```python
from build123d import *

# Parameters (mm, degrees)
Y_KSEKLIK_EKSTR_ZYON1_DEPTH = 40
RADYUS1_R                   = 1
RADYUS2_R                   = 0.3
RADYUS3_R                   = 1


with BuildPart() as part:
    # Çizim1 → Yükseklik-Ekstrüzyon1 (new body)
    with BuildSketch(Plane.XY):
        with BuildLine():
            Line((-8.6, -3.2), (-9.7, -3.2))
            Line((-9.7, -3.2), (-9.7, -3.7))
            Line((-9.7, -3.7), (-10, -3.7))
            Line((-10, -3.7), (-10, -10))
            Line((-10, -10), (-3.7, -10))
            Line((-3.7, -10), (-3.7, -9.7))
            Line((-3.7, -9.7), (-3.2, -9.7))
            Line((-3.2, -9.7), (-3.2, -8.6))
            Line((-3.2, -8.6), (-7.610050506, -8.6))
            Line((-7.610050506, -8.6), (-2.217957246, -3.20790674))
            ThreePointArc((-2.217957246, -3.20790674), (-1.299073648, -3.677282646), (-0.289258242, -3.889258242))
            Line((-0.289258242, -3.889258242), (0, -3.6))
            Line((0, -3.6), (0.289258242, -3.889258242))
            ThreePointArc((0.289258242, -3.889258242), (1.299073648, -3.677282646), (2.217957246, -3.20790674))
            Line((2.217957246, -3.20790674), (7.610050506, -8.6))
            Line((7.610050506, -8.6), (3.2, -8.6))
            Line((3.2, -8.6), (3.2, -9.7))
            Line((3.2, -9.7), (3.7, -9.7))
            Line((3.7, -9.7), (3.7, -10))
            Line((3.7, -10), (10, -10))
            Line((10, -10), (10, -3.7))
            Line((10, -3.7), (9.7, -3.7))
            Line((9.7, -3.7), (9.7, -3.2))
            Line((9.7, -3.2), (8.6, -3.2))
            Line((8.6, -3.2), (8.6, -7.610050506))
            Line((8.6, -7.610050506), (3.20790674, -2.217957246))
            ThreePointArc((3.20790674, -2.217957246), (3.677282646, -1.299073648), (3.889258242, -0.289258242))
            Line((3.889258242, -0.289258242), (3.6, 0))
            Line((3.6, 0), (3.889258242, 0.289258242))
            ThreePointArc((3.889258242, 0.289258242), (3.677282646, 1.299073648), (3.20790674, 2.217957246))
            Line((3.20790674, 2.217957246), (8.6, 7.610050506))
            Line((8.6, 7.610050506), (8.6, 3.2))
            Line((8.6, 3.2), (9.7, 3.2))
            Line((9.7, 3.2), (9.7, 3.7))
            Line((9.7, 3.7), (10, 3.7))
            Line((10, 3.7), (10, 10))
            Line((10, 10), (3.7, 10))
            Line((3.7, 10), (3.7, 9.7))
            Line((3.7, 9.7), (3.2, 9.7))
            Line((3.2, 9.7), (3.2, 8.6))
            Line((3.2, 8.6), (7.610050506, 8.6))
            Line((7.610050506, 8.6), (2.217957246, 3.20790674))
            ThreePointArc((2.217957246, 3.20790674), (1.299073648, 3.677282646), (0.289258242, 3.889258242))
            Line((0.289258242, 3.889258242), (0, 3.6))
            Line((0, 3.6), (-0.289258242, 3.889258242))
            ThreePointArc((-0.289258242, 3.889258242), (-1.299073648, 3.677282646), (-2.217957246, 3.20790674))
            Line((-2.217957246, 3.20790674), (-7.610050506, 8.6))
            Line((-7.610050506, 8.6), (-3.2, 8.6))
            Line((-3.2, 8.6), (-3.2, 9.7))
            Line((-3.2, 9.7), (-3.7, 9.7))
            Line((-3.7, 9.7), (-3.7, 10))
            Line((-3.7, 10), (-10, 10))
            Line((-10, 10), (-10, 3.7))
            Line((-10, 3.7), (-9.7, 3.7))
            Line((-9.7, 3.7), (-9.7, 3.2))
            Line((-9.7, 3.2), (-8.6, 3.2))
            Line((-8.6, 3.2), (-8.6, 7.610050506))
            Line((-8.6, 7.610050506), (-3.20790674, 2.217957246))
            ThreePointArc((-3.20790674, 2.217957246), (-3.677282646, 1.299073648), (-3.889258242, 0.289258242))
            Line((-3.889258242, 0.289258242), (-3.6, 0))
            Line((-3.6, 0), (-3.889258242, -0.289258242))
            ThreePointArc((-3.889258242, -0.289258242), (-3.677282646, -1.299073648), (-3.20790674, -2.217957246))
            Line((-3.20790674, -2.217957246), (-8.6, -7.610050506))
            Line((-8.6, -7.610050506), (-8.6, -3.2))
        make_face()
        with BuildLine():
            Line((1.967124912, -1.542860843), (2.333452378, -1.909188309))
            ThreePointArc((2.333452378, -1.909188309), (2.333452378, -2.333452378), (1.909188309, -2.333452378))
            Line((1.909188309, -2.333452378), (1.542860843, -1.967124912))
            ThreePointArc((1.542860843, -1.967124912), (0, -2.5), (-1.542860843, -1.967124912))
            Line((-1.542860843, -1.967124912), (-1.909188309, -2.333452378))
            ThreePointArc((-1.909188309, -2.333452378), (-2.333452378, -2.333452378), (-2.333452378, -1.909188309))
            Line((-2.333452378, -1.909188309), (-1.967124912, -1.542860843))
            ThreePointArc((-1.967124912, -1.542860843), (-2.5, 0), (-1.967124912, 1.542860843))
            Line((-1.967124912, 1.542860843), (-2.333452378, 1.909188309))
            ThreePointArc((-2.333452378, 1.909188309), (-2.333452378, 2.333452378), (-1.909188309, 2.333452378))
            Line((-1.909188309, 2.333452378), (-1.542860843, 1.967124912))
            ThreePointArc((-1.542860843, 1.967124912), (0, 2.5), (1.542860843, 1.967124912))
            Line((1.542860843, 1.967124912), (1.909188309, 2.333452378))
            ThreePointArc((1.909188309, 2.333452378), (2.333452378, 2.333452378), (2.333452378, 1.909188309))
            Line((2.333452378, 1.909188309), (1.967124912, 1.542860843))
            ThreePointArc((1.967124912, 1.542860843), (2.5, 0), (1.967124912, -1.542860843))
        make_face(mode=Mode.SUBTRACT)
    extrude(amount=Y_KSEKLIK_EKSTR_ZYON1_DEPTH)

    # Radyus1
    radyus1_edges = [part.edges().sort_by_distance(p)[0] for p in [
        (-2.217957246, -3.20790674, 20),
        (-3.20790674, -2.217957246, 20),
        (-3.20790674, 2.217957246, 20),
        (-2.217957246, 3.20790674, 20),
        (2.217957246, 3.20790674, 20),
        (3.20790674, 2.217957246, 20),
        (3.20790674, -2.217957246, 20),
        (2.217957246, -3.20790674, 20),
    ]]
    fillet(radyus1_edges, radius=RADYUS1_R)

    # Radyus2
    radyus2_edges = [part.edges().sort_by_distance(p)[0] for p in [
        (-7.610050506, -8.6, 20),
        (-8.6, -7.610050506, 20),
        (-8.6, 7.610050506, 20),
        (-7.610050506, 8.6, 20),
        (7.610050506, 8.6, 20),
        (8.6, 7.610050506, 20),
        (8.6, -7.610050506, 20),
        (7.610050506, -8.6, 20),
    ]]
    fillet(radyus2_edges, radius=RADYUS2_R)

    # Radyus3
    radyus3_edges = [part.edges().sort_by_distance(p)[0] for p in [
        (-10, -10, 20),
        (-10, 10, 20),
        (10, 10, 20),
        (10, -10, 20),
    ]]
    fillet(radyus3_edges, radius=RADYUS3_R)


solid = part.part
```
For this review, take the finished solid that the model builds, in its own axes (mm). A direction names the side the tool comes from. Round coordinates to 2 decimals unless told otherwise and drop trailing zeros. Loops run counter-clockwise (first coordinate to the right, second up) from the corner with the lowest first, then second, coordinate; pieces in that order, holes last.
(1) Mouldability with a two-part tool opening along X and no side actions: class faces 1 (the cylindrical face through (-2.5, 0, 19.7)), 2 (the flat face through (-6, -10, 20)), 3 (the flat face through (-10, 6, 20)), 4 (the cylindrical face through (3.774, -0.984, 19.72)) as released by +X, released by -X, zero draft, split by the parting line, or undercut.
Returned:
face 1: undercut
face 2: zero draft
face 3: released by -X
face 4: released by +X
(2) Clearance check with flat-ended pins moving along their axes: P1, Ø1.5, axis at x = 0.5, y = 5.5, coming from the -Z side; P2, Ø0.5, axis at x = -9.5, z = 23.5, coming from the +Y side. State where each tip first meets the part, or that it passes through.
Returned:
P1: passes through
P2: stops at y = 9.97
(3) We need section B-B (x = 5). Give the boundary of the cut face in (y, z).
Returned:
outline: (-10, 0) - (-8.6, 0) - (-8.6, 40) - (-10, 40) - close; (-5.99, 0) - (-4.01, 0) - (-4.01, 40) - (-5.99, 40) - close; (4.01, 0) - (5.99, 0) - (5.99, 40) - (4.01, 40) - close; (8.6, 0) - (10, 0) - (10, 40) - (8.6, 40) - close
(4) Tool access review of faces 5 (the flat face through (9, -3.2, 20)), 6 (the flat face through (-9, 3.2, 20)), 7 (the flat face through (10, 6, 20)), 8 (the flat face through (-5.95, 4.96, 19.72)), 9 (the flat face through (6, 10, 20)): name each direction out of +Z, -Z, +X, -X, +Y, -Y from which nothing blocks a thin tool from reaching the whole face with its end or side.
Returned:
face 5: +Z, -Z, +X
face 6: +Z, -Z, -X
face 7: +Z, -Z, +X, +Y, -Y
face 8: +Z, -Z
face 9: +Z, -Z, +X, -X, +Y
(5) We need section A-A (y = -6). Give the boundary of the cut face in (x, z).
Returned:
outline: (-10, 0) - (-8.6, 0) - (-8.6, 40) - (-10, 40) - close; (-6.99, 0) - (-5.01, 0) - (-5.01, 40) - (-6.99, 40) - close; (5.01, 0) - (6.99, 0) - (6.99, 40) - (5.01, 40) - close; (8.6, 0) - (10, 0) - (10, 40) - (8.6, 40) - close
(6) Wall thickness on line 1 along Y through (x, z) = (-4.75, 14); line 2 along Y through (x, z) = (6.25, 12); line 3 along X through (y, z) = (-3.25, 29.5): over which ranges is each line inside the solid? List them lowest first.
Returned:
line 1: y = -10 to -8.6, -5.74 to -3.76, 3.76 to 5.74, 8.6 to 10
line 2: y = -10 to -8.6, -7.24 to -5.26, 5.26 to 7.24, 8.6 to 10
line 3: x = -9.7 to -8.6, -4.24 to 4.24, 8.6 to 9.7
